The model under review builds one solid part; all positions refer to its coordinate system, in mm. Face numbers are marked on the shaded views. A direction names the side the tool comes from. Give positions to 0.01 mm unless a question says otherwise; leave off trailing zeros. Loops run counter-clockwise (first coordinate to the right, second up) from the corner with the lowest first, then second, coordinate; pieces in that order, holes last. Notation, with made-up numbers: M 4.5,-2.75 L 30.5,-2.75 A14 ccw 30.5,5.25 Z; hole C 21,5 d10. An arc over 180 degrees is marked long. Return JSON: item names as keys, results as strings.
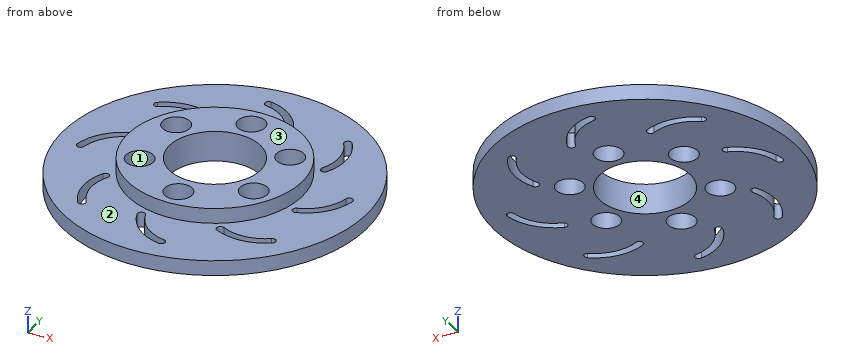
```python
from build123d import *

# Parameters (mm, degrees)
F0_R     = 11.5
F0_R_2   = 1.8
F0_R_3   = 6
F1_DEPTH = 4
F0_R_4   = 20
F2_DEPTH = 2
F4_DEPTH = 2.001


with BuildPart() as f1:
    # F0 (on Top) → F1 (new body)
    with BuildSketch(Plane.XY):
        Circle(F0_R)
        with Locations((-7.577722, -4.375)):
            Circle(F0_R_2, mode=Mode.SUBTRACT)
        with Locations((0, -8.75)):
            Circle(F0_R_2, mode=Mode.SUBTRACT)
        with Locations((7.577722, -4.375)):
            Circle(F0_R_2, mode=Mode.SUBTRACT)
        with Locations((-7.577722, 4.375)):
            Circle(F0_R_2, mode=Mode.SUBTRACT)
        Circle(F0_R_3, mode=Mode.SUBTRACT)
        with Locations((7.577722, 4.375)):
            Circle(F0_R_2, mode=Mode.SUBTRACT)
        with Locations((0, 8.75)):
            Circle(F0_R_2, mode=Mode.SUBTRACT)
    extrude(amount=F1_DEPTH)

    # F0 (on Top) → F2 (join)
    with BuildSketch(Plane.XY):
        Circle(F0_R_4)
        Circle(F0_R, mode=Mode.SUBTRACT)
    extrude(amount=F2_DEPTH)

    # F3 (on face) → F4 (cut, through all)
    with BuildSketch(Plane.XY.offset(2)):
        with BuildLine():
            ThreePointArc((-2.192977, 16.187632), (0.664228, 14.871151), (2.423816, 12.263358))
            ThreePointArc((2.423816, 12.263358), (3.055985, 11.946556), (3.372786, 12.578724))
            ThreePointArc((3.372786, 12.578724), (1.311876, 15.633091), (-2.034612, 17.175013))
            ThreePointArc((-2.034612, 17.175013), (-2.607485, 16.760505), (-2.192977, 16.187632))
        make_face()
        with BuildLine():
            ThreePointArc((6.957606, -10.3854), (6.286583, -10.608398), (6.509581, -11.279421))
            ThreePointArc((6.509581, -11.279421), (10.126628, -11.981901), (13.583256, -10.705881))
            ThreePointArc((13.583256, -10.705881), (13.695237, -10.007697), (12.997054, -9.895716))
            ThreePointArc((12.997054, -9.895716), (10.045812, -10.985172), (6.957606, -10.3854))
        make_face()
        with BuildLine():
            ThreePointArc((-2.423816, -12.263358), (-3.055985, -11.946556), (-3.372786, -12.578724))
            ThreePointArc((-3.372786, -12.578724), (-1.311876, -15.633091), (2.034612, -17.175013))
            ThreePointArc((2.034612, -17.175013), (2.607485, -16.760505), (2.192977, -16.187632))
            ThreePointArc((2.192977, -16.187632), (-0.664228, -14.871151), (-2.423816, -12.263358))
        make_face()
        with BuildLine():
            ThreePointArc((-10.3854, -6.957606), (-10.608398, -6.286583), (-11.279421, -6.509581))
            ThreePointArc((-11.279421, -6.509581), (-11.981901, -10.126628), (-10.705881, -13.583256))
            ThreePointArc((-10.705881, -13.583256), (-10.007697, -13.695237), (-9.895716, -12.997054))
            ThreePointArc((-9.895716, -12.997054), (-10.985172, -10.045812), (-10.3854, -6.957606))
        make_face()
        with BuildLine():
            ThreePointArc((-12.263358, 2.423816), (-11.946556, 3.055985), (-12.578724, 3.372786))
            ThreePointArc((-12.578724, 3.372786), (-15.633091, 1.311876), (-17.175013, -2.034612))
            ThreePointArc((-17.175013, -2.034612), (-16.760505, -2.607485), (-16.187632, -2.192977))
            ThreePointArc((-16.187632, -2.192977), (-14.871151, 0.664228), (-12.263358, 2.423816))
        make_face()
        with BuildLine():
            ThreePointArc((-6.957606, 10.3854), (-6.286583, 10.608398), (-6.509581, 11.279421))
            ThreePointArc((-6.509581, 11.279421), (-10.126628, 11.981901), (-13.583256, 10.705881))
            ThreePointArc((-13.583256, 10.705881), (-13.695237, 10.007697), (-12.997054, 9.895716))
            ThreePointArc((-12.997054, 9.895716), (-10.045812, 10.985172), (-6.957606, 10.3854))
        make_face()
        with BuildLine():
            ThreePointArc((10.3854, 6.957606), (10.608398, 6.286583), (11.279421, 6.509581))
            ThreePointArc((11.279421, 6.509581), (11.981901, 10.126628), (10.705881, 13.583256))
            ThreePointArc((10.705881, 13.583256), (10.007697, 13.695237), (9.895716, 12.997054))
            ThreePointArc((9.895716, 12.997054), (10.985172, 10.045812), (10.3854, 6.957606))
        make_face()
        with BuildLine():
            ThreePointArc((12.263358, -2.423816), (11.946556, -3.055985), (12.578724, -3.372786))
            ThreePointArc((12.578724, -3.372786), (15.633091, -1.311876), (17.175013, 2.034612))
            ThreePointArc((17.175013, 2.034612), (16.760505, 2.607485), (16.187632, 2.192977))
            ThreePointArc((16.187632, 2.192977), (14.871151, -0.664228), (12.263358, -2.423816))
        make_face()
    extrude(amount=-F4_DEPTH, mode=Mode.SUBTRACT)


solid = f1.part
```
1) The part is to be moulded in two halves that separate along Y. For the marked faces 3 and 4, say which applies: released by +Y, released by -Y, zero draft, split by the parting line, or undercut.
From the geometry:
{"face 3": "zero draft", "face 4": "undercut"}
2) Insertion check: pin 1 (1.5 mm diameter, centred on x = 15.5, y = 8.5, fed in from -Z); pin 2 (1 mm diameter, centred on y = 7, z = 2, fed in from -X); pin 3 (1.5 mm diameter, centred on y = 9.5, z = 1.5, fed in from +X). Each pin has a flat end and moves straight along its axis. Give the tip position at first contact, or say it passes through.
From the geometry:
{"pin 1": "z = 0", "pin 2": "x = -18.91", "pin 3": "x = 17.98"}
3) Consider section C-C on y = -8.75. Write out the cut boundary in (x, z).
From the geometry:
{"outline": "M -17.98,0 L -11.95,0 L -11.95,2 L -17.98,2 Z; M -10.95,0 L -1.8,0 L -1.8,4 L -7.46,4 L -7.46,2 L -10.95,2 Z; M 1.8,0 L 17.98,0 L 17.98,2 L 7.46,2 L 7.46,4 L 1.8,4 Z"}
4) Wall thickness on L1, parallel to Y at x = 0, z = 2.65; L2, parallel to Y at x = 8, z = 1.35; L3, parallel to Y at x = -6.5, z = 3.6: over which ranges is each line inside the solid? List them lowest first. Write a range as from..to.
From the geometry:
{"L1": "-11.5..-10.55, -6.95..-6, 6..6.95, 10.55..11.5", "L2": "-18.33..-11.82, -10.79..-6.12, -2.63..2.63, 6.12..18.33", "L3": "-9.49..-5.82, -2.93..2.93, 5.82..9.49"}
5) Consider section B-B on x = 0. Write out the cut boundary in (y, z).
From the geometry:
{"outline": "M -20,0 L -16.51,0 L -16.51,2 L -20,2 Z; M -15.36,0 L -10.55,0 L -10.55,4 L -11.5,4 L -11.5,2 L -15.36,2 Z; M -6.95,0 L -6,0 L -6,4 L -6.95,4 Z; M 6,0 L 6.95,0 L 6.95,4 L 6,4 Z; M 10.55,0 L 15.36,0 L 15.36,2 L 11.5,2 L 11.5,4 L 10.55,4 Z; M 16.51,0 L 20,0 L 20,2 L 16.51,2 Z"}
6) Consider section A-A on z = 2.5. Write out the cut boundary in (x, y) (3 decimals), then the cut area to 3 significant figures.
From the geometry:
{"outline": "C 0,0 d23; hole C -7.578,-4.375 d3.6; hole C -7.578,4.375 d3.6; hole C 0,0 d12; hole C 0,-8.75 d3.6; hole C 0,8.75 d3.6; hole C 7.578,-4.375 d3.6; hole C 7.578,4.375 d3.6", "area": "241 mm²"}
7) Consider section D-D on x = -15.5. Write out the cut boundary in (y, z).
From the geometry:
{"outline": "M -12.64,0 L -0.23,0 L -0.23,2 L -12.64,2 Z; M 1.46,0 L 12.64,0 L 12.64,2 L 1.46,2 Z"}
8) Tool access review of the marked faces 1 and 2: name each direction out of +Z, -Z, +X, -X, +Y, -Y from which nothing blocks a thin tool from reaching the whole face with its end or side.
From the geometry:
{"face 1": "+Z, -Z", "face 2": "+Z"}
